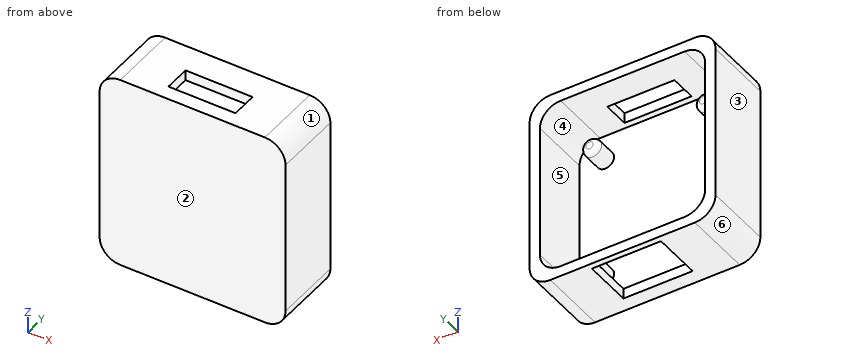
Autodesk Inventor part; units mm, degrees
ref_plane "YZ Plane" through (0, 0, 0) normal (1, 0, 0) x (0, 1, 0)
ref_plane "XZ Plane" through (0, 0, 0) normal (0, 1, 0) x (-1, 0, 0)
ref_plane "XY Plane" through (0, 0, 0) normal (0, 0, 1) x (1, 0, 0)
sketch "Sketch1" plane through (0, 0, 0) normal (0, 1, 0) x (-1, 0, 0)
  line L0 (0, 0) -> (22.86, 0)
  line L1 (22.86, 0) -> (22.86, -24.13)
  line L2 (22.86, -24.13) -> (0, -24.13)
  line L3 (0, -24.13) -> (0, 0)
  dimension "d0" = 24.13
  dimension "d1" = 22.86
extrude "Extrusion1" add sketch "Sketch1" along normal blind 8.5
sketch "Sketch2" plane through (0, 8.5, 0) normal (0, 1, 0) x (1, 0, 0)
  line L0 (-1.27, 1.27) -> (-21.59, 1.27)
  line L1 (-21.59, 1.27) -> (-21.59, 22.86)
  line L2 (-21.59, 22.86) -> (-1.27, 22.86)
  line L3 (-1.27, 22.86) -> (-1.27, 1.27)
  line L4 (-22.86, 0) -> (0, 0)
  line L5 (0, 24.13) -> (-22.86, 24.13)
  line L6 (0, 0) -> (0, 24.13)
  line L7 (-22.86, 24.13) -> (-22.86, 0)
  dimension "d4" = 21.59
  dimension "d5" = 20.32
  dimension "d6" = 1.27
  dimension "d7" = 1.27
  dimension "d8" = 1.27
  dimension "d9" = 1.27
extrude "Extrusion2" cut sketch "Sketch2" against normal blind 7.5 contours L0 L1 L2 L3
fillet "Fillet1" radius 2.54 4 edges at (-21.59, 4.75, -1.27) (-21.59, 4.75, -22.86) (-1.27, 4.75, -22.86) (-1.27, 4.75, -1.27)
sketch "Sketch3" plane through (0, 1, 0) normal (0, 1, 0) x (1, 0, 0)
  line L0 (-3.81, 1.27) -> (-19.05, 1.27)
  line L1 (-19.05, 22.86) -> (-3.81, 22.86)
  line L2 (-1.27, 20.32) -> (-1.27, 3.81)
  line L3 (-21.59, 3.81) -> (-21.59, 20.32)
  circle A0 centre (-18.415, 4.445) radius 1.0795
  circle A1 centre (-18.415, 19.685) radius 1.0795
  circle A2 centre (-4.445, 19.685) radius 1.0795
  circle A3 centre (-4.445, 4.445) radius 1.0795
  point P0 (0, 0)
  dimension "d13" = 13.97
  dimension "d14" = 15.24
  dimension "d15" = 13.97
  dimension "d16" = 15.24
  dimension "d17" = 3.175
  dimension "d19" = 3.175
  dimension "d20" = 3.175
  dimension "d21" = 3.175
  dimension "d22" = 3.175
  dimension "d23" = 3.175
  dimension "d24" = 2.159
extrude "Extrusion3" add sketch "Sketch3" along normal blind 3
fillet "Fillet2" radius 0.635 4 edges at (-19.4945, 4, -19.685) (-5.5245, 4, -19.685) (-19.4945, 4, -4.445) (-5.5245, 4, -4.445)
sketch "Sketch4" plane through (-22.86, 0, 0) normal (0, 0, 1) x (1, 0, 0)
  line L0 (7.305, 5.025) -> (15.555, 5.025)
  line L1 (15.555, 5.025) -> (15.555, 1.775)
  line L2 (15.555, 1.775) -> (7.305, 1.775)
  line L3 (7.305, 1.775) -> (7.305, 5.025)
  line L4 (0, 0) -> (0, 8.5)
  line L5 (22.86, 0) -> (22.86, 8.5)
  line L6 (19.05, 1) -> (3.81, 1)
  dimension "d28" = 8.25
  dimension "d29" = 3.25
  dimension "d30" = 7.305
  dimension "d31" = 7.305
  dimension "d32" = 0.775
extrude "Extrusion4" cut sketch "Sketch4" against normal up to surface (1.27 mm away)
sketch "Sketch5" plane through (0, 0, -24.13) normal (0, 0, -1) x (-1, 0, 0)
  line L0 (7.18, 7.775) -> (15.68, 7.775)
  line L1 (15.68, 7.775) -> (15.68, 1.775)
  line L2 (15.68, 1.775) -> (7.18, 1.775)
  line L3 (7.18, 1.775) -> (7.18, 7.775)
  line L4 (0, 0) -> (0, 8.5)
  line L5 (22.86, 0) -> (22.86, 8.5)
  line L6 (0, 0) -> (22.86, 0)
  line L7 (19.05, 1) -> (3.81, 1)
  dimension "d35" = 8.5
  dimension "d36" = 6
  dimension "d37" = 7.18
  dimension "d38" = 7.18
  dimension "d43" = 0.775
extrude "Extrusion5" cut sketch "Sketch5" against normal up to surface (1.27 mm away)
fillet "Fillet3" radius 2.54 4 edges at (0, 4.25, 0) (-22.86, 4.25, 0) (0, 4.25, -24.13) (-22.86, 4.25, -24.13)
equation "\"d6\" = d7"
equation "\"d8\" = d9"
equation "\"d30\" = d31"
equation "\"d37\" = d38"
properties part number "micro lipo case"
Work out the finished part from the listing and answer in its coordinate system (mm). Face numbers are marked on the shaded views. A direction names the side the tool comes from. Give positions to 0.01 mm unless a question says otherwise; leave off trailing zeros. Loops run counter-clockwise (first coordinate to the right, second up) from the corner with the lowest first, then second, coordinate; pieces in that order, holes last. Notation, with made-up numbers: (24.25, 68) - (78.25, 68) arc R13 cw to (78.25, 76) - close; hole circle Ø4 at (57.25, 0.25). An arc over 180 degrees is marked (long way). Answer in a Markdown table with one row per item. Add a question column.
Q1. Consider line 1 along X through (y, z) = (3, -11.5); line 2 along Y through (x, z) = (-13.5, -5.25); line 3 along X through (y, z) = (4, -3). Determine where each line is inside the solid, lowest interval first.
Q2. The part is cut by section C-C (z = -16.25). Determine the outline of the cut face in (x, y).
Q3. Each of these flat-tipped pins is pushed along its axis until it touches: P1, Ø1.4, axis at y = 5.5, z = -23.5, coming from the -X side; P2, Ø10, axis at x = -11, z = -11, coming from the +Y side; P3, Ø1, axis at y = 3, z = -0.5, coming from the +X side. Where does it stop, or does it pass through?
Q4. Determine the mould class of the marked faces 1, 2, 3 and 4 for opening direction X: released by +X, released by -X, zero draft, split by the parting line, or undercut.
Q5. A tool of negligible diameter and unlimited length cuts with its end or side. For the marked faces 5 and 6, from which of +Z, -Z, +X, -X, +Y, -Y can it reach the whole face along a straight path? Write none if from no direction.
Q6. The part is cut by section A-A (x = -13.5). Determine the outline of the cut face in (y, z) (3 decimals), and give its area (3 significant figures).
Q7. The part is cut by section D-D (y = 2.75). State how many separate pieces and enclosed holes the cut face has, and give its area (3 significant figures).
Q8. The part is cut by section B-B (y = 6.25). Determine the outline of the cut face in (x, z), and give its area (3 significant figures).
Solution:
| question | item | result |
|---|---|---|
| 1 | line 1 | x = -22.86 to -21.59, -1.27 to 0 |
| 1 | line 2 | y = 0 to 1 |
| 1 | line 3 | x = -22.86 to -21.46, -1.4 to 0 |
| 2 | outline | (-22.86, 0) - (0, 0) - (0, 8.5) - (-1.27, 8.5) - (-1.27, 1) - (-21.59, 1) - (-21.59, 8.5) - (-22.86, 8.5) - close |
| 3 | P1 | stops at x = -22.55 |
| 3 | P2 | stops at y = 1 |
| 3 | P3 | stops at x = -0.52 |
| 4 | face 1 | released by +X |
| 4 | face 2 | zero draft |
| 4 | face 3 | released by -X |
| 4 | face 4 | undercut |
| 5 | face 5 | +Y |
| 5 | face 6 | -Z, -X, +Y, -Y |
| 6 | outline | (0, -24.13) - (1.775, -24.13) - (1.775, -22.86) - (1, -22.86) - (1, -1.27) - (1.775, -1.27) - (1.775, 0) - (0, 0) - close; (5.025, -1.27) - (8.5, -1.27) - (8.5, 0) - (5.025, 0) - close; (7.775, -24.13) - (8.5, -24.13) - (8.5, -22.86) - (7.775, -22.86) - close |
| 6 | area | 31.4 mm² |
| 7 | separate pieces | 6 |
| 7 | enclosed holes | 0 |
| 7 | area | 106 mm² |
| 8 | outline | (-22.86, -21.59) arc R2.54 ccw to (-20.32, -24.13) - (-15.68, -24.13) - (-15.68, -22.86) - (-19.05, -22.86) arc R2.54 cw to (-21.59, -20.32) - (-21.59, -3.81) arc R2.54 cw to (-19.05, -1.27) - (-3.81, -1.27) arc R2.54 cw to (-1.27, -3.81) - (-1.27, -20.32) arc R2.54 cw to (-3.81, -22.86) - (-7.18, -22.86) - (-7.18, -24.13) - (-2.54, -24.13) arc R2.54 ccw to (0, -21.59) - (0, -2.54) arc R2.54 ccw to (-2.54, 0) - (-20.32, 0) arc R2.54 ccw to (-22.86, -2.54) - close |
| 8 | area | 102 mm² |
